Autodesk Inventor part; units mm, degrees
ref_plane "YZ Plane" through (0, 0, 0) normal (1, 0, 0) x (0, 1, 0)
ref_plane "XZ Plane" through (0, 0, 0) normal (0, 1, 0) x (-1, 0, 0)
ref_plane "XY Plane" through (0, 0, 0) normal (0, 0, 1) x (1, 0, 0)
sketch "Sketch1" plane through (0, 0, 0) normal (0, 0, 1) x (1, 0, 0)
  line L0 (-40, 5) -> (0, 5)
  line L1 (0, 5) -> (0, -5)
  line L2 (0, -5) -> (-40, -5)
  line L3 (-40, -5) -> (-40, 5)
  line L4 (-10, 35) -> (0, 35)
  line L5 (0, 35) -> (0, 5)
  line L6 (0, 5) -> (-10, 5)
  line L7 (-10, 5) -> (-10, 35)
  point P0 (0, 0)
  point P1 (0, 5)
  dimension "d0" = 10
  dimension "d1" = 40
  dimension "d2" = 40
extrude "Extrusion1" add sketch "Sketch1" along normal blind 40
sketch "Sketch2" plane through (-10, 5, 0) normal (-1, 0, 0) x (0, 0, 1)
  line L0 (8.5, 20) -> (11.5, 20) construction
  line L1 (8.5, 17) -> (11.5, 17)
  line L2 (11.5, 23) -> (8.5, 23)
  arc A0 (8.5, 23) -> (8.5, 17) centre (8.5, 20) ccw
  arc A1 (11.5, 17) -> (11.5, 23) centre (11.5, 20) ccw
  line L3 (0, 30) -> (0, 0)
  line L4 (0, 30) -> (40, 30)
  line L5 (20, 21.547) -> (20, 15) construction
  line L6 (31.5, 20) -> (28.5, 20) construction
  line L7 (31.5, 17) -> (28.5, 17)
  line L8 (28.5, 23) -> (31.5, 23)
  arc A2 (31.5, 17) -> (31.5, 23) centre (31.5, 20) ccw
  arc A3 (28.5, 23) -> (28.5, 17) centre (28.5, 20) ccw
  point P0 (0, -5)
  point P1 (10, 20)
  point P2 (20, 18.2735)
  point P3 (20, 30)
  point P4 (30, 20)
  dimension "d5" = 6
  dimension "d6" = 3
  dimension "d7" = 10
  dimension "d8" = 10
extrude "Extrusion2" cut sketch "Sketch2" against normal through all
sketch "Sketch3" plane through (-40, 5, 0) normal (0, 1, 0) x (1, 0, 0)
  line L0 (10, -8.5) -> (10, -11.5) construction
  line L1 (7, -8.5) -> (7, -11.5)
  line L2 (13, -11.5) -> (13, -8.5)
  arc A0 (13, -8.5) -> (7, -8.5) centre (10, -8.5) ccw
  arc A1 (7, -11.5) -> (13, -11.5) centre (10, -11.5) ccw
  line L3 (30, 0) -> (0, 0)
  line L4 (0, 0) -> (0, -40)
  line L5 (15.2557, -20) -> (9.287, -20) construction
  line L6 (10, -31.5) -> (10, -28.5) construction
  line L7 (7, -31.5) -> (7, -28.5)
  line L8 (13, -28.5) -> (13, -31.5)
  arc A2 (7, -31.5) -> (13, -31.5) centre (10, -31.5) ccw
  arc A3 (13, -28.5) -> (7, -28.5) centre (10, -28.5) ccw
  point P0 (40, 0)
  point P1 (10, -10)
  point P2 (12.2713, -20)
  point P3 (0, -20)
  point P4 (10, -30)
  dimension "d11" = 3
  dimension "d12" = 6
  dimension "d13" = 10
  dimension "d14" = 10
extrude "Extrusion3" cut sketch "Sketch3" against normal through all
chamfer "Chamfer1" distance 10 angle 45 1 edges at (-10, 5, 20)
fillet "Fillet1" radius 2 5 edges at (-10, 35, 20) (0, 35, 20) (0, -5, 20) (-40, -5, 20) (-40, 5, 20)
sketch "Sketch4" plane through (0, -3, 0) normal (1, 0, 0) x (0, 0, -1)
  line L0 (-40, 38) -> (-20, 38)
  line L1 (-20, 38) -> (-20, -2)
  line L2 (-20, -2) -> (-40, -2)
  line L3 (-40, -2) -> (-40, 38)
  line L4 (0, 38) -> (-40, 38)
  line L5 (-40, 0) -> (-40, 36)
  line L6 (-40, -2) -> (0, -2)
  line L7 (0, 0) -> (0, 36)
  point P0 (0, 3)
  dimension "d21" = 20
extrude "Extrusion4" cut sketch "Sketch4" against normal through all
equation "\"d2\" = d1"
properties part number "0008-10-030 Suport L" material "ABS Plastic"
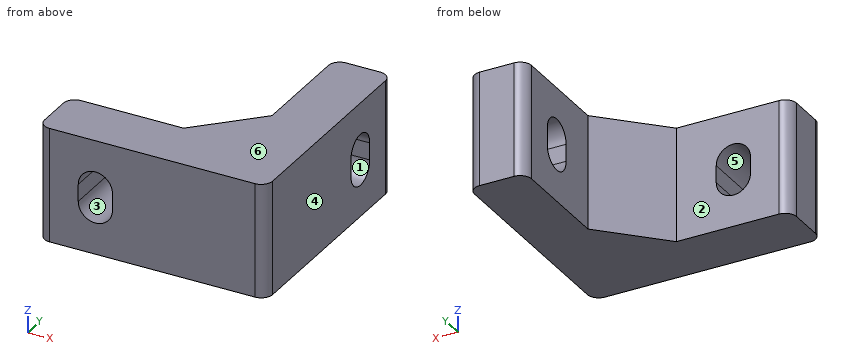
Could you check a few things on this model? Use its own coordinates, in mm. Face numbers are marked on the shaded views. A direction names the side the tool comes from. Coordinates: 2 decimals unless noted, no trailing zeros. Loops run counter-clockwise (first coordinate to the right, second up) from the corner with the lowest first, then second, coordinate; pieces in that order, holes last. Notation, with made-up numbers: M 26,22.5 L 53,22.5 A35 cw 53,57.5 Z; hole C -23.5,88.25 d9. An arc over 180 degrees is marked long. Put each result on its own line as item: value. Start each with the question number.
(1) Suppose I cut it at A-A on y = 0. Please give me the cut outline in (x, z), then the cut area to 3 significant figures.
(2) I need wall thicknesses on line 1 (X direction, y = 1.5, z = 11.25); line 2 (Y direction, x = -5, z = 8.5); line 3 (X direction, y = 17.5, z = 18.5). Which ranges of each line are inside material? Lowest first, please. Write a range as from..to.
(3) Will these pins go through, and if not, where does the flat tip stop? P1, Ø3, axis at y = 24.5, z = 17, coming from the -X side; P2, Ø5.5, axis at x = -32.5, z = 6.5, coming from the +Y side.
(4) Suppose I cut it at D-D on z = 4.25. Please give me the cut outline in (x, y), then the cut area to 3 significant figures.
(5) Thinking about a two-plate mould opening in X: for the marked faces 4, 5 and 6, which applies, pulls with the +X half, pulls with the -X half, needs draft (parallel to the pull), parting line crosses it, or undercut?
(6) For the marked faces 1, 2 and 3, which set-ups out of +Z, -Z, +X, -X, +Y, -Y let a thin tool reach every point of the face, with its end or its side?
(7) Suppose I cut it at C-C on y = 25. Please give me the cut outline in (x, z), then the cut area to 3 significant figures.
(8) Suppose I cut it at B-B on x = -30. Please give me the cut outline in (y, z).
Solutions:
1. outline: M -40,0 L 0,0 L 0,20 L -40,20 Z; hole M -33,8.5 A3 ccw -27,8.5 L -27,11.5 A3 ccw -33,11.5 Z
1. area: 754 mm2
2. line 1: x = -40..-33, -27..0
2. line 2: y = -5..22, 28..35
2. line 3: x = -10..0
3. P1: stops at x = -10
3. P2: stops at y = 5
4. outline: M -40,-3 A2 ccw -38,-5 L -2,-5 A2 ccw 0,-3 L 0,33 A2 ccw -2,35 L -8,35 A2 ccw -10,33 L -10,15 L -20,5 L -38,5 A2 ccw -40,3 Z
4. area: 746 mm2
5. face 4: pulls with the +X half
5. face 5: undercut
5. face 6: needs draft
6. face 1: +X, -X
6. face 2: +Z, -Z, -X, +Y
6. face 3: +Y, -Y
7. outline: M -10,0 L 0,0 L 0,5.5 L -10,5.5 Z; M -10,14.5 L 0,14.5 L 0,20 L -10,20 Z
7. area: 110 mm2
8. outline: M -5,0 L 5,0 L 5,5.5 L -5,5.5 Z; M -5,14.5 L 5,14.5 L 5,20 L -5,20 Z
